Input: part model. Units: mm. Frame: model coordinates. Coordinates: 2 decimals unless noted, no trailing zeros. Write each loop counter-clockwise with the first axis right and the second up, starting at its lowest first coordinate (ties: lowest second). Pieces come first, ordered by that corner, then holes.
from build123d import *

# Parameters (mm, degrees)
SKETCH_1_W        = 196
SKETCH_1_H        = 118
EXTRUDE_1_DEPTH   = 12
HOLE_WIZARD_M61_D = 6.647
HOLE_WIZARD_M62_D = 6.647
CHAMFER_1_SIZE    = 0.6765


with BuildPart() as part:
    # Эскиз1 → Бобышка-Вытянуть1 (new body)
    with BuildSketch(Plane.XY.offset(12)):
        Rectangle(SKETCH_1_W, SKETCH_1_H)
    extrude(amount=-EXTRUDE_1_DEPTH)

    # Отверстие с зазором M61 (through all)
    with Locations(Plane(origin=(0, 0, 0), x_dir=(-1, 0, 0), z_dir=(0, 0, -1))):
        with Locations((-66, -48)):
            Hole(HOLE_WIZARD_M61_D / 2)

    # Отверстие с зазором M62 (through all)
    with Locations(Plane.XY.offset(12)):
        with Locations((-66, 48), (-66, -48), (66, 48)):
            Hole(HOLE_WIZARD_M62_D / 2)

    # Фаска1
    chamfer_1_edges = [part.edges().sort_by_distance(p)[0] for p in [
        (62.6765, -48, 0),
        (62.6765, -48, 12),
        (69.3235, 48, 12),
        (69.3235, 48, 0),
        (-62.6765, -48, 12),
        (-62.6765, -48, 0),
        (-62.6765, 48, 12),
        (-62.6765, 48, 0),
    ]]
    chamfer(chamfer_1_edges, length=CHAMFER_1_SIZE)


solid = part.part
Item 1: Section query A-A, the plane y = 48. Return loops of the section in (x, z).
Item 2: Pull-direction query (X, two-part tool) for faces 1 (the face through (-1, -59, 6)), 2 (the face through (-98, -1, 6)), 3 (the face through (64.47, 45.05, 5.93)); classes: released by +X, released by -X, zero draft, split by the parting line, or undercut.
Item 3: Pin query (flat end, axial travel): pin 1 Ø8.5 at (x, y) = (66, -48) entering from +Z. Return the tip coordinate at first contact, or that it passes through.
Item 4: Material intervals for line 1 (Y direction, x = -66, z = 7.25); line 2 (X direction, y = -48.5, z = 5.5), sorted ascending.
Item 5: Section query B-B, the plane x = 66. Return loops of the section in (y, z).
The answers:
1. outline: (-98, 0) - (-70, 0) - (-69.32, 0.68) - (-69.32, 11.32) - (-70, 12) - (-98, 12) - close; (-62.68, 0.68) - (-62, 0) - (62, 0) - (62.68, 0.68) - (62.68, 11.32) - (62, 12) - (-62, 12) - (-62.68, 11.32) - close; (69.32, 0.68) - (70, 0) - (98, 0) - (98, 12) - (70, 12) - (69.32, 11.32) - close
2. face 1: zero draft
2. face 2: released by -X
2. face 3: undercut
3. pin 1: stops at z = 12
4. line 1: y = -59 to -51.32, -44.68 to 44.68, 51.32 to 59
4. line 2: x = -98 to -69.29, -62.71 to 62.71, 69.29 to 98
5. outline: (-59, 0) - (-52, 0) - (-51.32, 0.68) - (-51.32, 11.32) - (-52, 12) - (-59, 12) - close; (-44.68, 0.68) - (-44, 0) - (44, 0) - (44.68, 0.68) - (44.68, 11.32) - (44, 12) - (-44, 12) - (-44.68, 11.32) - close; (51.32, 0.68) - (52, 0) - (59, 0) - (59, 12) - (52, 12) - (51.32, 11.32) - close
